Autodesk Inventor part; units mm, degrees
ref_plane "YZ Plane" through (0, 0, 0) normal (1, 0, 0) x (0, 1, 0)
ref_plane "XZ Plane" through (0, 0, 0) normal (0, 1, 0) x (-1, 0, 0)
ref_plane "XY Plane" through (0, 0, 0) normal (0, 0, 1) x (1, 0, 0)
sketch "Sketch1" plane through (0, 0, 0) normal (0, 0, 1) x (1, 0, 0)
  line L0 (0, 0) -> (38.1, 0)
  line L1 (38.1, 0) -> (38.1, 38.1)
  line L2 (38.1, 38.1) -> (0, 38.1)
  line L3 (0, 38.1) -> (0, 0)
  dimension "d0" = 38.1
  dimension "d1" = 38.1
extrude "Extrusion1" add sketch "Sketch1" along normal blind 25.4
sketch "Sketch2" plane through (38.1, 0, 0) normal (1, 0, 0) x (0, 0, -1)
  line L0 (0, 0) -> (0, 38.1)
  circle A0 centre (-12.7, 12.7) radius 3.175
  line L1 (0, 0) -> (-25.4, 0)
  dimension "d5" = 12.7
  dimension "d6" = 6.35
  dimension "d18" = 12.7
extrude "Extrusion2" cut sketch "Sketch2" against normal through all
sketch "Sketch3" plane through (0, 0, 25.4) normal (0, 0, 1) x (1, 0, 0)
  line L0 (38.1, 38.1) -> (38.1, 0)
  line L1 (0, 38.1) -> (38.1, 38.1)
  line L2 (0, 38.1) -> (31.75, 38.1)
  line L3 (31.75, 38.1) -> (31.75, 19.05)
  line L4 (31.75, 19.05) -> (0, 19.05)
  line L5 (0, 19.05) -> (0, 38.1)
  dimension "d10" = 19.05
  dimension "d19" = 6.35
extrude "Extrusion3" cut sketch "Sketch3" against normal through all
sketch "Sketch5" plane through (0, 0, 0) normal (0, -1, 0) x (1, 0, 0)
  line L0 (38.1, 25.4) -> (0, 25.4)
  line L1 (0, 0) -> (0, 25.4)
  circle A0 centre (12.7, 12.7) radius 2.0735
  dimension "d20" = 12.7
  dimension "d21" = 12.7
extrude "Extrusion5" cut sketch "Sketch5" against normal through all
properties part number "ArmPivotBlock"
Model file for the job. Use its own axes, mm. A direction names the side the tool comes from. Give positions to 0.01 mm unless a question says otherwise; leave off trailing zeros. Loops run counter-clockwise (first coordinate to the right, second up) from the corner with the lowest first, then second, coordinate; pieces in that order, holes last. Notation, with made-up numbers: (-36.75, 80) - (-25.75, 80) arc R26 cw to (-25.75, 103) - close; hole circle Ø1 at (29.5, -13). An arc over 180 degrees is marked (long way). One line per item, written item: value. Start each with the question number.
1. Slice it at D-D (x = 27). List the corners of the cut face in (y, z) (3 decimals), plus the area to 3 significant figures.
2. Pin check, flat tips, straight feed: pin 1 (10 mm diameter, centred on y = 12.7, z = 12.7, fed in from +X); pin 2 (6 mm diameter, centred on y = 23.5, z = 7, fed in from -X); pin 3 (5.5 mm diameter, centred on x = 12.7, z = 12.7, fed in from +Y). Stop position of each tip, or through.
3. Slice it at A-A (y = 12.7). List the corners of the cut face in (x, z) (3 decimals).
4. Probe L1, parallel to X at y = 6, z = 12.5; L2, parallel to Z at x = 12.7, y = 16.55; L3, parallel to Y at x = 15, z = 15. List the from-to ranges inside material, lowest first. Write a range as from..to.
5. Which spindle directions (+Z, -Z, +X, -X, +Y, -Y) get a long thin tool onto all of the face, cutting with end or side? Do faces 5 (the flat face through (35, 38.1, 13)), 6 (the flat face through (16, 19.05, 13)). Say none if no direction does.
6. Pull direction X, two halves, no side cores. Call faces 1 (the flat face through (38.1, 19, 13)), 2 (the cylindrical face through (10.63, 5.08, 12.79)), 3 (the flat face through (19, 11, 25.4)), 4 (the flat face through (31.75, 29, 13)): pulls with the +X half, pulls with the -X half, needs draft (parallel to the pull), parting line crosses it, or undercut.
7. Slice it at C-C (z = 12.7). Give the number of separate pieces and of enclosed holes in the cut face, plus the area to 3 significant figures.
Solution:
1. outline: (0, 0) - (19.05, 0) - (19.05, 25.4) - (0, 25.4) - close; hole circle Ø6.35 at (12.7, 12.7)
1. area: 452 mm^2
2. pin 1: stops at x = 38.1
2. pin 2: stops at x = 31.75
2. pin 3: stops at y = 19.05
3. outline: (0, 0) - (38.1, 0) - (38.1, 9.525) - (0, 9.525) - close; (0, 15.875) - (38.1, 15.875) - (38.1, 25.4) - (0, 25.4) - close
4. L1: x = 0..10.64, 14.76..38.1
4. L2: z = 0..10.63, 14.77..25.4
4. L3: y = 0..10.51, 14.89..19.05
5. face 5: +Z, -Z, +X, -X, +Y
5. face 6: +Z, -Z, -X, +Y
6. face 1: pulls with the +X half
6. face 2: undercut
6. face 3: needs draft
6. face 4: pulls with the -X half
7. separate pieces: 4
7. enclosed holes: 0
7. area: 552 mm^2
